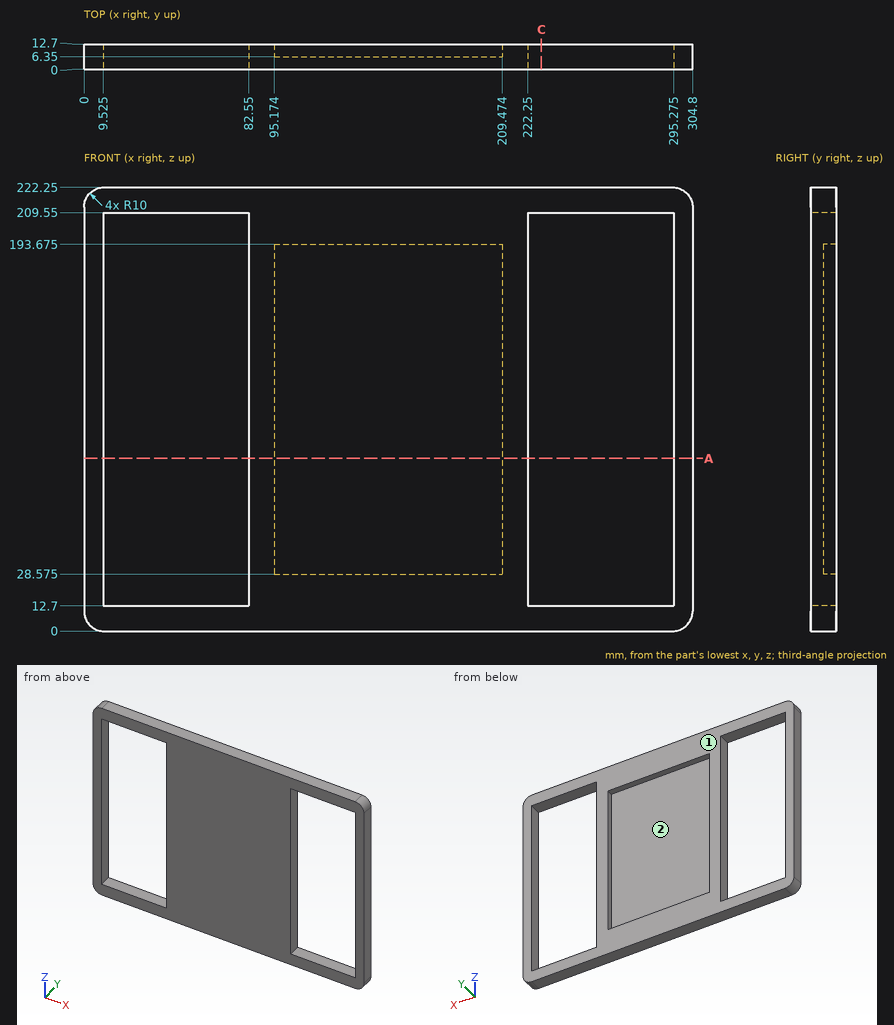
Geometry check sheet. Reference: drawing and pictorial views, mm from the part's lowest x, y, z. Coordinates: 2 decimals unless noted, no trailing zeros. Order: outer loops, then holes, each group sorted by start corner. A loop starts at its lowest first (then second) coordinate and runs counter-clockwise, first axis right, second up. Notation, with made-up numbers: M 42.25,48 L 63.25,48 A19 cw 63.25,78 Z; hole C 51,84.5 d8. An arc over 180 degrees is marked long. Write each question's results on one line, items separated by ' | '. Start each with the question number.
1. Material ranges on probe 1 along Z at (x, y) = (270.5, 5); probe 2 along Y at (x, z) = (101.5, 82), recorded low to high.
2. Mould release check, pull along Z, two halves, no side actions. Record for the marked faces 1 and 2: +Z half, -Z half, draft (parallel to the pull), parting line (faces both ways), or undercut.
3. Cross-section at A-A on z = 86.5. State how many separate pieces and enclosed holes the cut face has, and give its area (3 significant figures).
4. Cross-section at C-C on x = 229. Record the cut outline in (y, z).
5. Go/stop test with a flat-tipped pin: P1, Ø2, axis at x = 200.5, z = 160.5, coming from the +Y side. Record where the tip stops, or that it passes through.
Checks:
1) probe 1: z = 0 to 12.7, 209.55 to 222.25 | probe 2: y = 0 to 6.35
2) face 1: draft | face 2: undercut
3) separate pieces: 3 | enclosed holes: 0 | area: 1,290 mm²
4) outline: M 0,0 L 12.7,0 L 12.7,12.7 L 0,12.7 Z; M 0,209.55 L 12.7,209.55 L 12.7,222.25 L 0,222.25 Z
5) P1: stops at y = 6.35
